Design review of the part built by this model. Coordinates are the model's own, in mm. Face numbers are marked on the shaded views. Round coordinates to 2 decimals unless told otherwise and drop trailing zeros. Order: outer loops, then holes, each group sorted by start corner. A loop starts at its lowest first (then second) coordinate and runs counter-clockwise, first axis right, second up. Notation, with made-up numbers: (37, 48.5) - (64, 48.5) arc R6 cw to (64, 58.5) - close; hole circle Ø3 at (58.5, 41). An arc over 180 degrees is marked (long way). Use CSV: the item, a comma, the result in double quotes.
from build123d import *

# Parameters (mm, degrees)
SKICA2_W                 = 50
SKICA2_H                 = 4.2
P_IDAT_VYSUNUT_M2_DEPTH  = 0.4
SKICA3_R                 = 1.75
P_IDAT_VYSUNUT_M3_DEPTH  = 1.5
SKICA5_R                 = 1.9
P_IDAT_VYSUNUT_M5_DEPTH  = 2
ZKOSEN_2_SIZE            = 1.5
SKICA7_W                 = 1
SKICA7_H                 = 5
ODEBRAT_VYSUNUT_M1_DEPTH = 3.5
SKICA8_W                 = 4.2
SKICA8_H                 = 22.9
P_IDAT_VYSUNUT_M6_DEPTH  = 0.4
SKICA9_R                 = 1.75
P_IDAT_VYSUNUT_M7_DEPTH  = 1.5
SKICA10_R                = 1.9
P_IDAT_VYSUNUT_M8_DEPTH  = 2
ZKOSEN_3_SIZE            = 1.5
SKICA12_W                = 5
SKICA12_H                = 1
ODEBRAT_VYSUNUT_M2_DEPTH = 3.5


with BuildPart() as part:
    # Skica2 → Přidat vysunutím2 (new body)
    with BuildSketch(Plane.XY):
        Rectangle(SKICA2_W, SKICA2_H)
    extrude(amount=P_IDAT_VYSUNUT_M2_DEPTH)

    # Skica3 → Přidat vysunutím3 (add)
    with BuildSketch(Plane.XY.offset(0.4)):
        with Locations((-16, -0.2)):
            Circle(SKICA3_R)
        with Locations((16, 0)):
            Circle(SKICA3_R)
    extrude(amount=P_IDAT_VYSUNUT_M3_DEPTH)

    # Skica5 → Přidat vysunutím5 (add)
    with BuildSketch(Plane.XY.offset(1.9)):
        with Locations((-16, -0.2)):
            Circle(SKICA5_R)
        with Locations((16, 0)):
            Circle(SKICA5_R)
    extrude(amount=P_IDAT_VYSUNUT_M5_DEPTH)

    # Zkosení2
    zkosen_2_edges = [part.edges().sort_by_distance(p)[0] for p in [
        (-17.9, -0.2, 3.9),
        (14.1, 0, 3.9),
    ]]
    chamfer(zkosen_2_edges, length=ZKOSEN_2_SIZE)

    # Skica7 → Odebrat vysunutím1 (cut)
    with BuildSketch(Plane.XY.offset(3.9)):
        with Locations((-16, -0.2)):
            Rectangle(SKICA7_W, SKICA7_H)
        with Locations((16, 0)):
            Rectangle(SKICA7_W, SKICA7_H)
    extrude(amount=-ODEBRAT_VYSUNUT_M1_DEPTH, mode=Mode.SUBTRACT)

    # Skica8 → Přidat vysunutím6 (add)
    with BuildSketch(Plane(origin=(0, 0, 0), x_dir=(-1, 0, 0), z_dir=(0, 0, -1))):
        with Locations((0, -13.55)):
            Rectangle(SKICA8_W, SKICA8_H)
    extrude(amount=-P_IDAT_VYSUNUT_M6_DEPTH)

    # Skica9 → Přidat vysunutím7 (add)
    with BuildSketch(Plane.XY.offset(0.4)):
        with Locations((0, -16)):
            Circle(SKICA9_R)
    extrude(amount=P_IDAT_VYSUNUT_M7_DEPTH)

    # Skica10 → Přidat vysunutím8 (add)
    with BuildSketch(Plane.XY.offset(1.9)):
        with Locations((0, -16)):
            Circle(SKICA10_R)
    extrude(amount=P_IDAT_VYSUNUT_M8_DEPTH)

    # Zkosení3
    zkosen_3_edges = [part.edges().sort_by_distance(p)[0] for p in [
        (-1.9, -16, 3.9),
    ]]
    chamfer(zkosen_3_edges, length=ZKOSEN_3_SIZE)

    # Skica12 → Odebrat vysunutím2 (cut)
    with BuildSketch(Plane.XY.offset(3.9)):
        with Locations((0, -16)):
            Rectangle(SKICA12_W, SKICA12_H)
    extrude(amount=-ODEBRAT_VYSUNUT_M2_DEPTH, mode=Mode.SUBTRACT)


solid = part.part
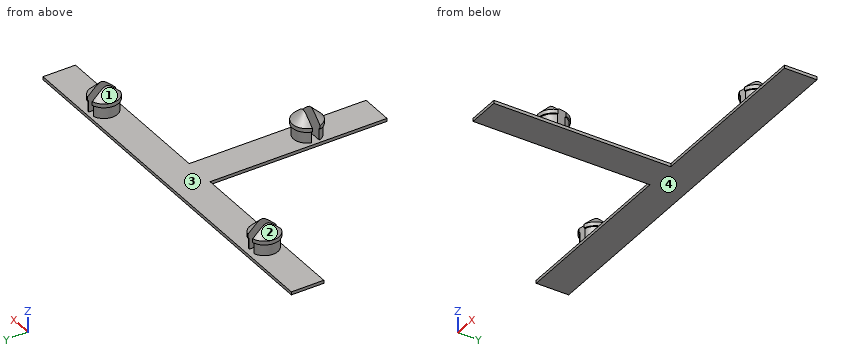
1) We need section B-B (y = -3.75). Give the boundary of the cut face in (x, z), then the cut area to 3 significant figures.
Data:
outline,"(-2.1, 0) - (2.1, 0) - (2.1, 0.4) - (-2.1, 0.4) - close"
area,"1.68 mm2"
2) Insertion check: pin 1 Ø1.7 at (y, z) = (-0.5, 2.5) entering from -X; pin 2 Ø1.5 at (x, z) = (2, 2.5) entering from -Y; pin 3 Ø1.7 at (y, z) = (0, 2.5) entering from +X. Each pin has a flat end and moves straight along its axis. Give the tip position at first contact, or say it passes through.
Data:
pin 1,"stops at x = -17.9"
pin 2,"stops at y = -17.43"
pin 3,"stops at x = 17.9"
3) The part is to be moulded in two halves that separate along X. For the marked faces 1, 2, 3 and 4, say which applies: +X half, -X half, draft (parallel to the pull), parting line (faces both ways), or undercut.
Data:
face 1,"undercut"
face 2,"-X half"
face 3,"undercut"
face 4,"draft"
4) We need section A-A (z = 3.25). Give the boundary of the cut face in (x, y).
Data:
outline,"(-16.5, -1.12) - (-16.5, 0.72) arc R1.05 ccw to start; (-15.5, -1.12) arc R1.05 ccw to (-15.5, 0.72) - close; (-0.92, -16.5) arc R1.05 ccw to (0.92, -16.5) - close; (-0.92, -15.5) - (0.92, -15.5) arc R1.05 ccw to start; (15.5, -0.92) - (15.5, 0.92) arc R1.05 ccw to start; (16.5, -0.92) arc R1.05 ccw to (16.5, 0.92) - close"
5) To check wall thickness, follow L1, parallel to X at y = -1.25, z = 0.6; L2, parallel to Z at x = -11, y = -1.25; L3, parallel to X at y = -0.25, z = 2.5. State the ranges of each line that lie inside material, in increasing order. Write a range as from..to.
Data:
L1,"x = -17.4..-16.5, -15.5..-14.6, 14.78..15.5, 16.5..17.22"
L2,"z = 0..0.4"
L3,"x = -17.8..-16.5, -15.5..-14.2, 14.22..15.5, 16.5..17.78"
